```python
from build123d import *

# Parameters (mm, degrees)
SKETCH1_W           = 135
SKETCH1_H           = 6
BOSS_EXTRUDE1_DEPTH = 80
SKETCH2_W           = 12.04
SKETCH2_H           = 6
CUT_EXTRUDE1_DEPTH  = 26


with BuildPart() as part:
    # Sketch1 → Boss-Extrude1 (new body)
    with BuildSketch(Plane.XY):
        Rectangle(SKETCH1_W, SKETCH1_H)
    extrude(amount=BOSS_EXTRUDE1_DEPTH)

    # Sketch2 → Cut-Extrude1 (cut)
    with BuildSketch(Plane.XY.offset(80)):
        with Locations((31.48, 0)):
            Rectangle(SKETCH2_W, SKETCH2_H)
        Polygon((-34.075898385, 3), (-37.54, -3), (-51.442594482, -3), (-47.978492867, 3), align=None)
    extrude(amount=-CUT_EXTRUDE1_DEPTH, mode=Mode.SUBTRACT)


solid = part.part
```
CAD build for the part. Positions are in the model's coordinates, mm. A direction names the side the tool comes from. Round coordinates to 2 decimals unless told otherwise and drop trailing zeros. Write each loop counter-clockwise with the first axis right and the second up, starting at its lowest first coordinate (ties: lowest second). Pieces come first, ordered by that corner, then holes. Notation, with made-up numbers: (-10, 69) - (14, 69) arc R25 ccw to (14, 103) - close; hole circle Ø7 at (67.5, 85.5). An arc over 180 degrees is marked (long way). Return JSON: item names as keys, results as strings. Group by question number.
Item 1: Probe probe 1 along X at (y, z) = (-1.55, 66.5); probe 2 along X at (y, z) = (-0.7, 76.5); probe 3 along Y at (x, z) = (-35.5, 71). List the from-to ranges inside material, lowest first.
Item 2: Mould opens along X. For faces 1 (the face through (-67.5, 0, 39)), 2 (the face through (52, 0, 80)), 3 (the face through (37.5, 0, 67)) say: +X half, -X half, draft (parallel to the pull), parting line (faces both ways), or undercut.
Item 3: Flat gauge pins, fed straight in: pin 1 Ø1.8 at (x, y) = (-41, -1.5) entering from +Z; pin 2 Ø2 at (x, y) = (45.5, 2.5) entering from -Z. Where does each tip first touch, or does it go through?
Item 4: 3-axis set-ups, long thin cutter, end or side, ignore diameter. For faces 4 (the face through (31, 0, 54)), 5 (the face through (-49.735, -0.042, 67.182)), 6 (the face through (-43, 0, 54)): which of +Z, -Z, +X, -X, +Y, -Y reach the whole face in a straight line?
Item 5: Band-saw the part on B-B on y = -0.7. List the corners of the cut face in (x, z).
Item 6: Band-saw the part on C-C on x = 31.5. List the corners of the cut face in (y, z).
Item 7: Band-saw the part on A-A on z = 67. List the corners of the cut face in (x, y), plus the area to 3 significant figures.
Resolved:
{
 "1": {"probe 1": "x = -67.5 to -50.61, -36.7 to 25.46, 37.5 to 67.5", "probe 2": "x = -67.5 to -50.11, -36.21 to 25.46, 37.5 to 67.5", "probe 3": "y = -3 to 0.53"},
 "2": {"face 1": "-X half", "face 2": "draft", "face 3": "undercut"},
 "3": {"pin 1": "stops at z = 54", "pin 2": "stops at z = 0"},
 "4": {"face 4": "+Z, +Y, -Y", "face 5": "+Z, -Y", "face 6": "+Z"},
 "5": {"outline": "(-67.5, 0) - (67.5, 0) - (67.5, 80) - (37.5, 80) - (37.5, 54) - (25.46, 54) - (25.46, 80) - (-36.21, 80) - (-36.21, 54) - (-50.11, 54) - (-50.11, 80) - (-67.5, 80) - close"},
 "6": {"outline": "(-3, 0) - (3, 0) - (3, 54) - (-3, 54) - close"},
 "7": {"outline": "(-67.5, -3) - (-51.44, -3) - (-47.98, 3) - (-67.5, 3) - close; (-37.54, -3) - (25.46, -3) - (25.46, 3) - (-34.08, 3) - close; (37.5, -3) - (67.5, -3) - (67.5, 3) - (37.5, 3) - close", "area": "654 mm²"}
}
